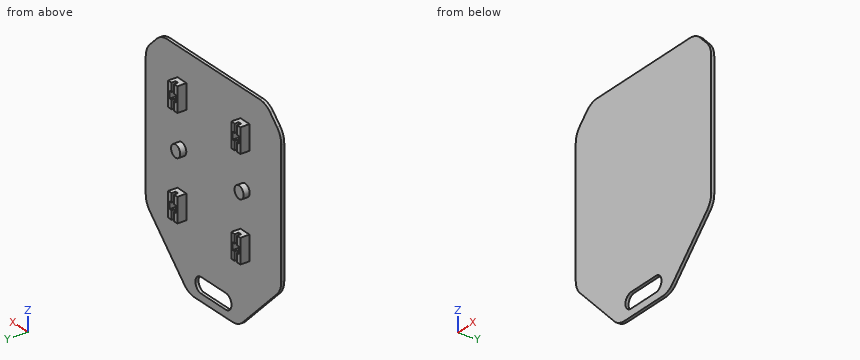
```python
from build123d import *

# Parameters (mm, degrees)
BODY_DEPTH          = 6.35
HANDLE_DEPTH        = 6.35
FILLET1_R           = 40
FILLET2_R           = 40
SKETCH3_W           = 25.4
SKETCH3_H           = 50.8
BOSS_EXTRUDE2_DEPTH = 19.05
SKETCH4_W           = 17.78
SKETCH4_H           = 14.7447
CUT_EXTRUDE1_DEPTH  = 17.78
SKETCH5_W           = 6.35
SKETCH5_H           = 18.02765
CUT_EXTRUDE2_DEPTH  = 8.5725
SKETCH6_R           = 12.7
BOSS_EXTRUDE3_DEPTH = 12.7


with BuildPart() as part:
    # Sketch1 → Body (new body)
    with BuildSketch(Plane(origin=(0, 0, 0), x_dir=(1, 0, 0), z_dir=(0, 1, 0))):
        Polygon((0, 0), (294, 0), (336.996020767, 43.003978862), (336.996020767, 337.003978862), (217, 456.999999629), (77, 456.999999629), (-42.996020767, 337.003978862), (-42.996020767, 43.003978862), align=None)
    extrude(amount=BODY_DEPTH)

    # Sketch2 → Handle (cut)
    with BuildSketch(Plane(origin=(0, 6.35, 0), x_dir=(1, 0, 0), z_dir=(0, 1, 0))):
        with BuildLine():
            Line((112.35, 441.799999629), (181.65, 441.799999629))
            ThreePointArc((181.65, 441.799999629), (197.5, 425.949999629), (181.65, 410.099999629))
            Line((181.65, 410.099999629), (112.35, 410.099999629))
            ThreePointArc((112.35, 410.099999629), (96.5, 425.949999629), (112.35, 441.799999629))
        make_face()
    extrude(amount=-HANDLE_DEPTH, mode=Mode.SUBTRACT)

    # Fillet1
    fillet1_edges = [part.edges().sort_by_distance(p)[0] for p in [
        (77, 3.175, -456.999999629),
        (217, 3.175, -456.999999629),
    ]]
    fillet(fillet1_edges, radius=FILLET1_R)

    # Fillet2
    fillet2_edges = [part.edges().sort_by_distance(p)[0] for p in [
        (-42.996020767, 3.175, -43.003978862),
        (-42.996020767, 3.175, -337.003978862),
        (336.996020767, 3.175, -337.003978862),
        (336.996020767, 3.175, -43.003978862),
        (294, 3.175, 0),
        (0, 3.175, 0),
    ]]
    fillet(fillet2_edges, radius=FILLET2_R)

    # Sketch3 → Boss-Extrude2 (add)
    with BuildSketch(Plane(origin=(0, 6.35, 0), x_dir=(1, 0, 0), z_dir=(0, 1, 0))):
        with Locations((235.396020767, 295.035436367)):
            Rectangle(SKETCH3_W, SKETCH3_H)
        with Locations((58.603979233, 295.035436367)):
            Rectangle(SKETCH3_W, SKETCH3_H)
        with Locations((235.396020767, 84.970353145)):
            Rectangle(SKETCH3_W, SKETCH3_H)
        with Locations((58.603979233, 84.970353145)):
            Rectangle(SKETCH3_W, SKETCH3_H)
    extrude(amount=BOSS_EXTRUDE2_DEPTH)

    # Sketch4 → Cut-Extrude1 (cut)
    with BuildSketch(Plane(origin=(0, 25.4, 0), x_dir=(1, 0, 0), z_dir=(0, 1, 0))):
        with Locations((58.603979233, 295.035436367)):
            Rectangle(SKETCH4_W, SKETCH4_H)
        with Locations((235.396020767, 295.035436367)):
            Rectangle(SKETCH4_W, SKETCH4_H)
        with Locations((58.603979233, 84.970353145)):
            Rectangle(SKETCH4_W, SKETCH4_H)
        with Locations((235.396020767, 84.970353145)):
            Rectangle(SKETCH4_W, SKETCH4_H)
    extrude(amount=-CUT_EXTRUDE1_DEPTH, mode=Mode.SUBTRACT)

    # Sketch5 → Cut-Extrude2 (cut)
    with BuildSketch(Plane(origin=(0, 25.4, 0), x_dir=(1, 0, 0), z_dir=(0, 1, 0))):
        with Locations((58.603979233, 101.356528145)):
            Rectangle(SKETCH5_W, SKETCH5_H)
        with Locations((58.603979233, 311.421611367)):
            Rectangle(SKETCH5_W, SKETCH5_H)
        with Locations((58.603979233, 278.649261367)):
            Rectangle(SKETCH5_W, SKETCH5_H)
        with Locations((235.396020767, 278.649261367)):
            Rectangle(SKETCH5_W, SKETCH5_H)
        with Locations((235.396020767, 311.421611367)):
            Rectangle(SKETCH5_W, SKETCH5_H)
        with Locations((58.603979233, 68.584178145)):
            Rectangle(SKETCH5_W, SKETCH5_H)
        with Locations((235.396020767, 68.584178145)):
            Rectangle(SKETCH5_W, SKETCH5_H)
        with Locations((235.396020767, 101.356528145)):
            Rectangle(SKETCH5_W, SKETCH5_H)
    extrude(amount=-CUT_EXTRUDE2_DEPTH, mode=Mode.SUBTRACT)

    # Sketch6 → Boss-Extrude3 (add)
    with BuildSketch(Plane(origin=(0, 6.35, 0), x_dir=(1, 0, 0), z_dir=(0, 1, 0))):
        with Locations(Location((58.1, 190.5, 0), (0, 0, 90))):
            Circle(SKETCH6_R)
        with Locations(Location((235.9, 190.5, 0), (0, 0, 90))):
            Circle(SKETCH6_R)
    extrude(amount=BOSS_EXTRUDE3_DEPTH)


solid = part.part
```
Design review of the part built by this model. Coordinates are the model's own, in mm. Coordinates: 2 decimals unless noted, no trailing zeros. Order: outer loops, then holes, each group sorted by start corner. A loop starts at its lowest first (then second) coordinate and runs counter-clockwise, first axis right, second up. Notation, with made-up numbers: (-4.5, -36.75) - (42.5, -36.75) arc R32 ccw to (42.5, -8.75) - close; hole circle Ø11 at (10, 12). An arc over 180 degrees is marked (long way). Answer in a Markdown table with one row per item.
(1) Consider section A-A on y = 12.5. Give the number of separate pieces and of enclosed holes in the cut face, plus the area to 3 significant figures.
Checked values:
| item | result |
|---|---|
| separate pieces | 6 |
| enclosed holes | 4 |
| area | 5,130 mm^2 |
(2) Consider section D-D on x = 32.5. State the section outline as (y, z) points, plus the area to 3 significant figures.
Checked values:
| item | result |
|---|---|
| outline | (0, -412.5) - (6.35, -412.5) - (6.35, 0) - (0, 0) - close |
| area | 2,620 mm^2 |
(3) Consider section B-B on z = -425.95. State the section outline as (x, y) points.
Checked values:
| item | result |
|---|---|
| outline | (45.95, 0) - (96.5, 0) - (96.5, 6.35) - (45.95, 6.35) - close; (197.5, 0) - (248.05, 0) - (248.05, 6.35) - (197.5, 6.35) - close |
(4) Consider section C-C on z = -190.5. State the section outline as (x, y) points.
Checked values:
| item | result |
|---|---|
| outline | (-43, 0) - (337, 0) - (337, 6.35) - (248.6, 6.35) - (248.6, 19.05) - (223.2, 19.05) - (223.2, 6.35) - (70.8, 6.35) - (70.8, 19.05) - (45.4, 19.05) - (45.4, 6.35) - (-43, 6.35) - close |
(5) Wall thickness on line 1 along X through (y, z) = (20.5, -281); line 2 along Z through (x, y) = (51.5, 8); line 3 along X through (y, z) = (13, -275): over which ranges is each line inside the solid? List them lowest first. Write a range as from..to.
Checked values:
| item | result |
|---|---|
| line 1 | 45.9..55.43, 61.78..71.3, 222.7..232.22, 238.57..248.1 |
| line 2 | -320.44..-302.41, -287.66..-269.64, -201.35..-179.65, -110.37..-92.34, -77.6..-59.57 |
| line 3 | 45.9..71.3, 222.7..248.1 |
(6) Clearance check with flat-ended pins moving along their axes: pin 1 (5.5 mm diameter, centred on x = 61, y = 20, fed in from -Z); pin 2 (2 mm diameter, centred on x = 136.5, z = -394, fed in from -Y); pin 3 (4.5 mm diameter, centred on y = 21.5, z = -315, fed in from +X); pin 4 (5 mm diameter, centred on x = 79, z = -305, fed in from +Y). State where each tip first meets the part, or that it passes through.
Checked values:
| item | result |
|---|---|
| pin 1 | z = -320.44 |
| pin 2 | y = 0 |
| pin 3 | x = 248.1 |
| pin 4 | y = 6.35 |
